from build123d import *

# Parameters (mm, degrees)
F0_W        = 5.8
F0_H        = 7.3
F0_W_2      = 14
F0_H_2      = 9.8
F0_W_3      = 6
F1_DEPTH    = 6
F2_DEPTH    = 10
F3_R        = 1.8
F4_DEPTH    = 46
F5_T4_DEPTH = 50.6794044701


# Not quite as in the source:
# - a fillet or chamfer that OpenCascade refuses, or shapes differently, is made with other operations: its cross-section is extruded or revolved along the edge and cut away or added


with BuildPart() as f1:
    # F0 (on Top) → F1 (new body)
    with BuildSketch(Plane.XY):
        with Locations((49.0534804702, 31.8385251075)):
            Rectangle(F0_W, F0_H)
        with Locations((49.0534804702, 19.3385251075)):
            Rectangle(F0_W, F0_H)
        with Locations((-108.8465195298, 12.3885251075)):
            Rectangle(F0_W_2, F0_H_2)
        with Locations((43.1534804702, 31.8385251075)):
            Rectangle(F0_W_3, F0_H)
        with Locations((43.1534804702, 19.3385251075)):
            Rectangle(F0_W_3, F0_H)
        Polygon((-99.8465195298, 7.6040180652), (-99.8465195298, 33.7885251075), (-115.8465195298, 33.7885251075), (-115.8465195298, 31.2885251075), (-115.8465195298, 23.7885251075), (-101.8465195298, 23.7885251075), (-101.8465195298, 17.2885251075), (-101.8465195298, 7.4885251075), align=None)
        Polygon((40.1534804702, 28.1885251075), (40.1534804702, 35.4885251075), (-99.8465195298, 33.7885251075), (-99.8465195298, 7.6040180652), (40.1534804702, 15.6885251075), (40.1534804702, 22.9885251075), align=None)
        Polygon((-90.6591936946, 19.0157179874), (-90.6591936946, 26.0108020157), (32.8437909484, 26.0108020157), (32.8437909484, 23.3903356981), align=None, mode=Mode.SUBTRACT)
    extrude(amount=F1_DEPTH)

    # F0 (on Top) → F2 (join)
    with BuildSketch(Plane.XY):
        Polygon((-99.8465195298, 7.6040180652), (-99.8465195298, 33.7885251075), (-115.8465195298, 33.7885251075), (-115.8465195298, 31.2885251075), (-115.8465195298, 23.7885251075), (-101.8465195298, 23.7885251075), (-101.8465195298, 17.2885251075), (-101.8465195298, 7.4885251075), align=None)
        with Locations((-108.8465195298, 12.3885251075)):
            Rectangle(F0_W_2, F0_H_2)
    extrude(amount=F2_DEPTH)

    # F3 (on Front) → F4 (cut)
    with BuildSketch(Plane.XZ):
        with Locations((-109.3465195298, 5.7222666219)):
            Circle(F3_R)
    extrude(amount=-F4_DEPTH, mode=Mode.SUBTRACT)

    # F5: fillet of radius 5 on 1 edges, made by hand


with BuildPart() as f5_tool2:
    # F5_s3 → F5_t4 (new body)
    with BuildSketch(Plane.XZ.offset(-46.0359738214)):
        with BuildLine():
            ThreePointArc((-94.9475400442, 6), (-98.1098177044, 7.1270166538), (-99.8465195298, 10))
            Line((-99.8465195298, 10), (-99.8465195298, 6))
            Line((-99.8465195298, 6), (-94.9475400442, 6))
        make_face()
    extrude(amount=F5_T4_DEPTH)

    split(bisect_by=Plane(origin=(-0.4249488426, 34.9957870373, 0), x_dir=(0, 0, 1), z_dir=(0.012141962, -0.9999262837, 0)), keep=Keep.TOP)

    split(bisect_by=Plane(origin=(-0.7694930518, 13.3253674816, 0), x_dir=(0, 0, 1), z_dir=(-0.0576504367, 0.9983368305, 0)), keep=Keep.TOP)


with BuildPart() as f1_1:
    add(f1.part)

    # F5_t1: union F5_tool2
    add(f5_tool2.part)


solid = f1_1.part
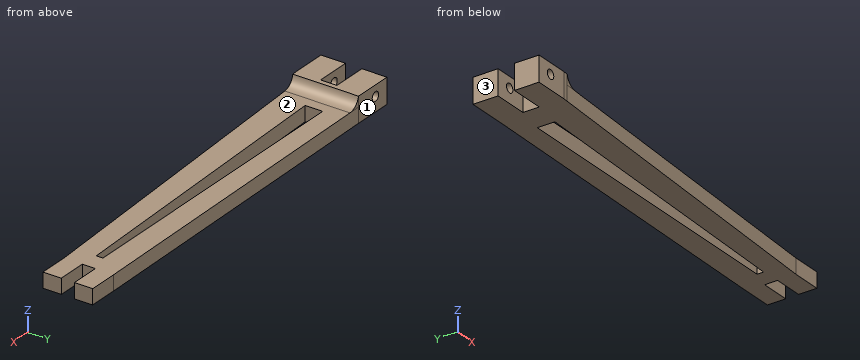
Can you work these out from the model? Positions are in its coordinate system, mm. Face numbers are marked on the shaded views. A direction names the side the tool comes from. Give positions to 0.01 mm unless a question says otherwise; leave off trailing zeros. Write each loop counter-clockwise with the first axis right and the second up, starting at its lowest first coordinate (ties: lowest second). Pieces come first, ordered by that corner, then holes. Notation, with made-up numbers: (89.25, 84) -> (146.25, 84) arc R27 ccw to (146.25, 118) -> close; hole circle Ø3 at (28, -27). An arc over 180 degrees is marked (long way). Answer as a JSON object with one key per item and string values. Group by question number.
Item 1: Suppose I cut it at A-A (x = 9). Please give me the cut outline in (y, z), plus the area to 3 significant figures.
Item 2: Please list where these lines run through material, in increasing order: line 1 (X direction, y = 28, z = 5.75); line 2 (Z direction, x = -33.5, y = 28); line 3 (X direction, y = 24.25, z = 2.5). Write a range as [from, to].
Item 3: Suppose I cut it at B-B (y = 12). Please give me the cut outline in (x, z), plus the area to 3 significant figures.
Item 4: Suppose I cut it at C-C (x = -85). Please give me the cut outline in (y, z), plus the area to 3 significant figures.
Item 5: I'm going to push flat-ended pins straight in: P1, Ø2.5, axis at y = 26, z = 2, coming from the +X side; P2, Ø3, axis at x = 45, z = 3.5, coming from the -Y side; P3, Ø14, axis at x = 2, y = 23, coming from the +Z side. Where does each tip first touch, or does it pass through?
Item 6: For the marked faces 1, 2 and 3, which set-ups out of +Z, -Z, +X, -X, +Y, -Y let a thin tool reach every point of the face, with its end or its side?
Item 7: Suppose I cut it at D-D (x = 38.5). Please give me the cut outline in (y, z).
Findings:
{
 "1": {"outline": "(13.89, 0) -> (22.55, 0) -> (22.55, 6) -> (13.89, 6) -> close; (26.01, 0) -> (35.11, 0) -> (35.11, 6) -> (26.01, 6) -> close", "area": "107 mm²"},
 "2": {"line 1": "x = [-115.85, -111.15], [-107.55, 40.15]", "line 2": "z = [0, 6]", "line 3": "x = [-115.85, -90.66], [32.84, 40.15]"},
 "3": {"outline": "(-115.85, 0) -> (-23.72, 0) -> (-23.72, 6) -> (-94.95, 6) arc R5 cw to (-99.85, 10) -> (-115.85, 10) -> close; hole circle Ø3.6 at (-109.35, 5.72)", "area": "612 mm²"},
 "4": {"outline": "(8.46, 0) -> (19.22, 0) -> (19.22, 6) -> (8.46, 6) -> close; (26.01, 0) -> (33.97, 0) -> (33.97, 6) -> (26.01, 6) -> close", "area": "112 mm²"},
 "5": {"P1": "stops at x = 40.15", "P2": "stops at y = 15.69", "P3": "stops at z = 6"},
 "6": {"face 1": "+Z, -Z, -X, +Y", "face 2": "+Z, +X, +Y, -Y", "face 3": "+Z, -Z, -X, +Y, -Y"},
 "7": {"outline": "(15.59, 0) -> (35.47, 0) -> (35.47, 6) -> (15.59, 6) -> close"}
}
